from build123d import *

# Parameters (mm, degrees)
F0_W          = 254
F0_H          = 660.4
F1_DEPTH      = 203.2
F3_DEPTH      = 50.8
F3_DEPTH_BACK = 203.2
F4_R          = 101.6
F6_DEPTH      = 660.4
F8_DEPTH      = 1302.3629254774
F9_R          = 190.5
F9_R_2        = 101.6
F10_DEPTH     = 1302.3629254774


with BuildPart() as f1:
    # F0 (on Top) → F1 (new body)
    with BuildSketch(Plane.XY):
        with Locations((-127, 0)):
            Rectangle(F0_W, F0_H)
    extrude(amount=-F1_DEPTH)

    # F2 (on face) → F3 (join, two sides)
    with BuildSketch(Plane.XY) as f3_sk:
        Polygon((-254, 330.2), (-254, 457.2), (-1397, 457.2), (-1397, -457.2), (-254, -457.2), (-254, -330.2), align=None)
        with BuildLine():
            ThreePointArc((-1016, -228.6), (-1244.6, 0), (-1016, 228.6))
            Line((-1016, 228.6), (-762, 228.6))
            ThreePointArc((-762, 228.6), (-533.4, 0), (-762, -228.6))
            Line((-762, -228.6), (-1016, -228.6))
        make_face(mode=Mode.SUBTRACT)
    extrude(amount=F3_DEPTH)
    extrude(f3_sk.sketch, amount=-F3_DEPTH_BACK)

    # F4
    f4_edges = [f1.edges().sort_by_distance(p)[0] for p in [
        (-254, -457.2, -76.2),
        (-254, 457.2, -76.2),
        (-1397, 457.2, -76.2),
        (-1397, -457.2, -76.2),
    ]]
    fillet(f4_edges, radius=F4_R)

    # F5 (on face) → F6 (join)
    with BuildSketch(Plane.XZ.offset(330.2)):
        Polygon((945.8729460134, -546.1), (0, 0), (-87.2836349805, -151.1796904555), (858.5893110329, -697.2796904555), align=None)
    extrude(amount=-F6_DEPTH)

    # F7 (on face) → F8 (cut, through all)
    with BuildSketch(Plane(origin=(0, 0, 0), x_dir=(0.8660254038, 0, -0.5), z_dir=(0.5, 0, 0.8660254038))):
        with BuildLine():
            ThreePointArc((1092.2, -1.051e-06), (995.4866587762, -233.4866595194), (762, -330.2))
            Line((762, -330.2), (1092.2, -330.2))
            Line((1092.2, -330.2), (1092.2, -1.051e-06))
        make_face()
        with BuildLine():
            ThreePointArc((762, 330.2), (995.4866595194, 233.4866587762), (1092.2, -1.051e-06))
            Line((1092.2, -1.051e-06), (1092.2, 330.2))
            Line((1092.2, 330.2), (762, 330.2))
        make_face()
    extrude(amount=-F8_DEPTH, mode=Mode.SUBTRACT)

    # F9 (on face) → F10 (cut, through all)
    with BuildSketch(Plane(origin=(0, 0, 0), x_dir=(0.8660254038, 0, -0.5), z_dir=(0.5, 0, 0.8660254038))):
        with Locations((762, 0)):
            Circle(F9_R)
        with Locations((254, 0)):
            Circle(F9_R_2)
    extrude(amount=-F10_DEPTH, mode=Mode.SUBTRACT)


solid = f1.part
Work out the finished part from the listing and answer in its coordinate system (mm). A direction names the side the tool comes from. Round coordinates to 2 decimals unless told otherwise and drop trailing zeros. Write each loop counter-clockwise with the first axis right and the second up, starting at its lowest first coordinate (ties: lowest second). Pieces come first, ordered by that corner, then holes.
1) Straight lines are drawn through the part: line 1 (X direction, y = -14.5, z = 16); line 2 (Z direction, x = -1266, y = 372); line 3 (X direction, y = 206, z = -151). For each, find the intervals that lie inside material, in ascending order.
2) A tool of negligible diameter and unlimited length cuts with its end or side. For faces 1 (the flat face through (167, -330.2, -206)), 2 (the flat face through (-553, 108, -203.2)), 3 (the cylindrical face through (-533.455, 5.027, -74.422)), 4 (the flat face through (-1397, 5, -74)), 5 (the cylindrical face through (258.2, -38.9, -248.5)), from which of +Z, -Z, +X, -X, +Y, -Y can it reach the whole face along a straight path? Write none if from no direction.
3) A cutting plane is placed at D-D (y = -264). Give the vertices of the cut face in (x, z), plus the area to 3 significant figures.
4) The mould has two halves that part along X. Classify faces 6 (the flat face through (479.558, -4.623, -276.873)), 7 (the flat face through (167, 330.2, -206)), 8 (the flat face through (-887, -228.6, -74)): pulls with the +X half, pulls with the -X half, needs draft (parallel to the pull), parting line crosses it, or undercut.
5) Given pin 1 Ø12 at (y, z) = (314.5, -406.5) entering from +X; pin 2 Ø6 at (x, y) = (-391, 17) entering from -Z; pin 3 Ø1.3 at (y, z) = (-23, -202) entering from +X, each flat-ended and moving along its own axis, determine where each tip first touches the part or whether it passes through.
6) A cutting plane is placed at B-B (z = -21). Give the vertices of the cut face in (x, y), plus the area to 3 significant figures.
7) A cutting plane is placed at C-C (y = 0). Give the vertices of the cut face in (x, z) (3 decimals), plus the area to 3 significant figures.
8) A cutting plane is placed at A-A (x = -839.5). Give the vertices of the cut face in (y, z).
Completed:
1. line 1: x = -1397 to -1244.14, -533.86 to -254
1. line 2: z = -203.2 to 50.8
1. line 3: x = -1397 to -1115.11, -662.89 to 261.54
2. face 1: +Z, -Z, +X, -Y
2. face 2: -Z, -X, +Y, -Y
2. face 3: +Z, -Z
2. face 4: +Z, -Z, -X, +Y, -Y
2. face 5: none
3. outline: (-1397, -203.2) - (0, -203.2) - (0, -201.57) - (744.39, -631.35) - (831.67, -480.17) - (0, 0) - (-254, 0) - (-254, 50.8) - (-1397, 50.8) - close
3. area: 501,000 mm2
4. face 6: pulls with the +X half
4. face 7: needs draft
4. face 8: undercut
5. pin 1: stops at x = 714.47
5. pin 2: stops at z = -203.2
5. pin 3: stops at x = 351
6. outline: (-1397, -355.6) arc R101.6 ccw to (-1295.4, -457.2) - (-355.6, -457.2) arc R101.6 ccw to (-254, -355.6) - (-254, -330.2) - (36.37, -330.2) - (36.37, 330.2) - (-254, 330.2) - (-254, 355.6) arc R101.6 ccw to (-355.6, 457.2) - (-1295.4, 457.2) arc R101.6 ccw to (-1397, 355.6) - close; hole (-1016, -228.6) - (-762, -228.6) arc R228.6 ccw to (-762, 228.6) - (-1016, 228.6) arc R228.6 ccw to start
6. area: 948,000 mm2
7. outline: (-1397, -203.2) - (-1244.6, -203.2) - (-1244.6, 50.8) - (-1397, 50.8) - close; (-533.4, -203.2) - (0, -203.2) - (0, -201.573) - (44.699, -227.38) - (131.982, -76.2) - (0, 0) - (-254, 0) - (-254, 50.8) - (-533.4, 50.8) - close; (220.675, -328.98) - (407.65, -436.93) - (494.934, -285.75) - (307.959, -177.8) - close; (737.606, -627.43) - (858.589, -697.28) - (945.873, -546.1) - (824.889, -476.25) - close
7. area: 241,000 mm2
8. outline: (-457.2, -203.2) - (-228.6, -203.2) - (-228.6, 50.8) - (-457.2, 50.8) - close; (228.6, -203.2) - (457.2, -203.2) - (457.2, 50.8) - (228.6, 50.8) - close
